Verification items for this drawing (mm, ordinates from the low corner). Coordinates: 2 decimals unless noted, no trailing zeros. Order: outer loops, then holes, each group sorted by start corner. A loop starts at its lowest first (then second) coordinate and runs counter-clockwise, first axis right, second up.
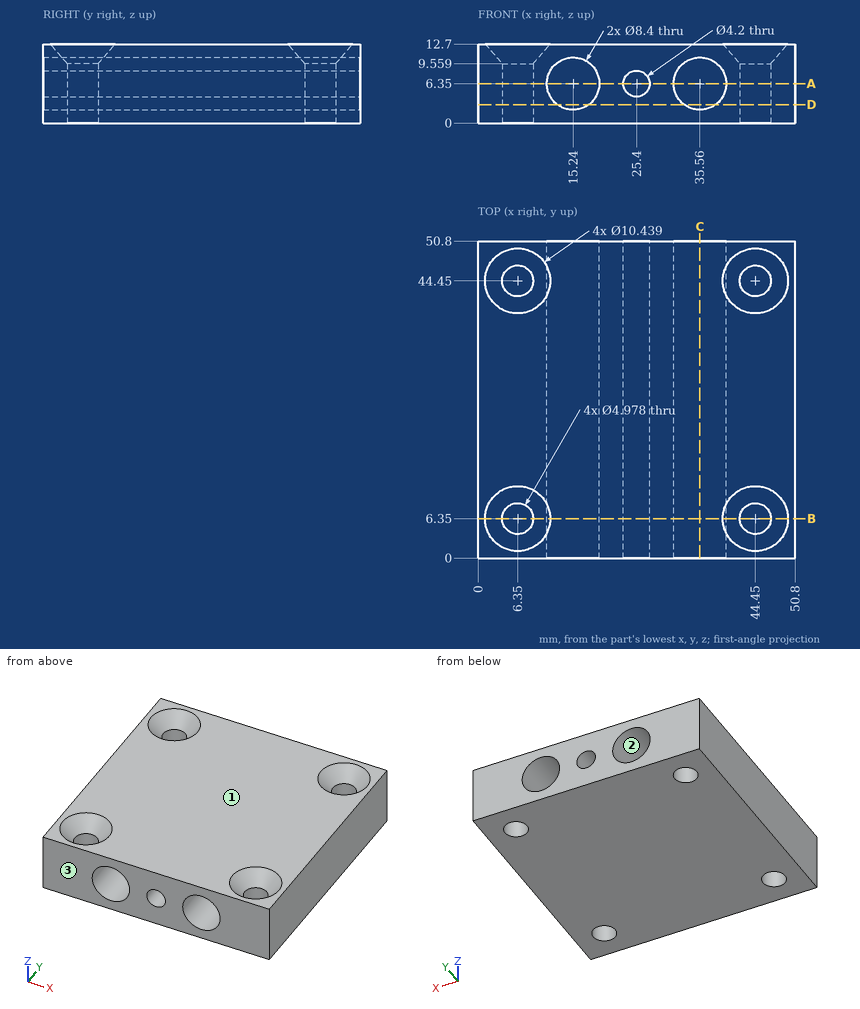
(1) Cross-section at A-A (z = 6.35). Enter the section's corners in (x, y), and give its area (3 significant figures).
Filled in:
outline: (0, 0) - (11.04, 0) - (11.04, 50.8) - (0, 50.8) - close; (19.44, 0) - (23.3, 0) - (23.3, 50.8) - (19.44, 50.8) - close; (27.5, 0) - (31.36, 0) - (31.36, 50.8) - (27.5, 50.8) - close; (39.76, 0) - (50.8, 0) - (50.8, 50.8) - (39.76, 50.8) - close; hole circle Ø4.98 at (6.35, 6.35); hole circle Ø4.98 at (6.35, 44.45); hole circle Ø4.98 at (44.45, 6.35); hole circle Ø4.98 at (44.45, 44.45)
area: 1,440 mm2
(2) Release check for a two-part mould opening along Z. For the marked faces 1, 2 and 3 record: +Z half, -Z half, draft (parallel to the pull), parting line (faces both ways), or undercut.
Filled in:
face 1: +Z half
face 2: undercut
face 3: draft
(3) Cross-section at B-B (y = 6.35). Enter the section's corners in (x, z).
Filled in:
outline: (0, 0) - (3.86, 0) - (3.86, 9.56) - (1.13, 12.7) - (0, 12.7) - close; (8.84, 0) - (41.96, 0) - (41.96, 9.56) - (39.23, 12.7) - (11.57, 12.7) - (8.84, 9.56) - close; (46.94, 0) - (50.8, 0) - (50.8, 12.7) - (49.67, 12.7) - (46.94, 9.56) - close; hole circle Ø8.4 at (15.24, 6.35); hole circle Ø4.2 at (25.4, 6.35); hole circle Ø8.4 at (35.56, 6.35)
(4) Go/stop test with a flat-tipped pin: P1, Ø5, axis at x = 15.24, z = 6.35, coming from the -Y side. Record where the tip stops, or that it passes through.
Filled in:
P1: passes through
(5) Thickness scan on probe 1 along Y at (x, z) = (6.35, 5.25); probe 2 along X at (y, z) = (48, 6.5) (1 decimal); probe 3 along X at (y, z) = (35, 8.25) (1 decimal). Record the ranges inside material, lowest first.
Filled in:
probe 1: y = 0 to 3.86, 8.84 to 41.96, 46.94 to 50.8
probe 2: x = 0 to 11, 19.4 to 23.3, 27.5 to 31.4, 39.8 to 50.8
probe 3: x = 0 to 11.5, 19 to 24.5, 26.3 to 31.8, 39.3 to 50.8
(6) Cross-section at D-D (z = 3). Enter the section's corners in (x, y).
Filled in:
outline: (0, 0) - (12.71, 0) - (12.71, 50.8) - (0, 50.8) - close; (17.77, 0) - (33.03, 0) - (33.03, 50.8) - (17.77, 50.8) - close; (38.09, 0) - (50.8, 0) - (50.8, 50.8) - (38.09, 50.8) - close; hole circle Ø4.98 at (6.35, 6.35); hole circle Ø4.98 at (6.35, 44.45); hole circle Ø4.98 at (44.45, 6.35); hole circle Ø4.98 at (44.45, 44.45)
(7) Cross-section at C-C (x = 35.56). Enter the section's corners in (y, z).
Filled in:
outline: (0, 0) - (50.8, 0) - (50.8, 2.15) - (0, 2.15) - close; (0, 10.55) - (50.8, 10.55) - (50.8, 12.7) - (0, 12.7) - close
